Could you check a few things on this model? Use its own coordinates, in mm. A direction names the side the tool comes from. Coordinates: 2 decimals unless noted, no trailing zeros. Write each loop counter-clockwise with the first axis right and the second up, starting at its lowest first coordinate (ties: lowest second). Pieces come first, ordered by that corner, then holes.
```python
from build123d import *

# Parameters (mm, degrees)
ESQUISSE1_R          = 1
BASE_EXTRUSION_DEPTH = 1.2


with BuildPart() as part:
    # Esquisse1 → Base-Extrusion (new body)
    with BuildSketch(Plane.XY):
        with BuildLine():
            Line((-1, -11.406248288), (-1, -15.467708298))
            ThreePointArc((-1, -15.467708298), (-2.37520157, -15.316932379), (-3.731481481, -15.044136597))
            ThreePointArc((-3.731481481, -15.044136597), (-4.825271875, -14.335239515), (-5.25, -13.102957681))
            Line((-5.25, -13.102957681), (-5.25, -12.716407865))
            ThreePointArc((-5.25, -12.716407865), (-5.532204997, -11.692112826), (-6.299180328, -10.956878965))
            ThreePointArc((-6.299180328, -10.956878965), (0, 13.95), (6.299180328, -10.956878965))
            ThreePointArc((6.299180328, -10.956878965), (5.532204997, -11.692112826), (5.25, -12.716407865))
            Line((5.25, -12.716407865), (5.25, -13.102957681))
            ThreePointArc((5.25, -13.102957681), (4.825271875, -14.335239515), (3.731481481, -15.044136597))
            ThreePointArc((3.731481481, -15.044136597), (2.37520157, -15.316932379), (1, -15.467708298))
            Line((1, -15.467708298), (1, -11.406248288))
            ThreePointArc((1, -11.406248288), (0, 11.45), (-1, -11.406248288))
        make_face()
        with Locations((3.25, -13.102957681)):
            Circle(ESQUISSE1_R, mode=Mode.SUBTRACT)
        with Locations((-3.25, -13.102957681)):
            Circle(ESQUISSE1_R, mode=Mode.SUBTRACT)
    extrude(amount=BASE_EXTRUSION_DEPTH)


solid = part.part
```
1. I want a section at A-A on z = 0.4. Please give me the cut outline in (x, y), plus the area to 3 significant figures.
Verdict:
outline: (-6.3, -10.96) arc R2 cw to (-5.25, -12.72) - (-5.25, -13.1) arc R2 ccw to (-3.73, -15.04) arc R15.5 ccw to (-1, -15.47) - (-1, -11.41) arc R11.45 cw (long way) to (1, -11.41) - (1, -15.47) arc R15.5 ccw to (3.73, -15.04) arc R2 ccw to (5.25, -13.1) - (5.25, -12.72) arc R2 cw to (6.3, -10.96) arc R13.25 ccw (long way) to start; hole circle Ø2 at (-3.25, -13.1); hole circle Ø2 at (3.25, -13.1)
area: 156 mm2
2. If we mould it in two halves opening along X, with no side actions, what happens to faces 1 (the face through (1, -13, 1)), 2 (the face through (-3.38, -12.11, 0.59)), 3 (the face through (-2.36, -15.32, 0.59)), 4 (the face through (2.394, -15.314, 0.592))? For each: pulls with the +X half, pulls with the -X half, needs draft (parallel to the pull), parting line crosses it, or undercut.
Verdict:
face 1: undercut
face 2: undercut
face 3: pulls with the -X half
face 4: pulls with the +X half
3. I want a section at D-D on x = -3.25. Please give me the cut outline in (y, z).
Verdict:
outline: (-15.16, 0) - (-14.1, 0) - (-14.1, 1.2) - (-15.16, 1.2) - close; (-12.1, 0) - (-10.98, 0) - (-10.98, 1.2) - (-12.1, 1.2) - close; (10.98, 0) - (13.55, 0) - (13.55, 1.2) - (10.98, 1.2) - close
4. I want a section at C-C on x = 8.75. Please give me the cut outline in (y, z).
Verdict:
outline: (-9.25, 0) - (-7.39, 0) - (-7.39, 1.2) - (-9.25, 1.2) - close; (7.39, 0) - (10.65, 0) - (10.65, 1.2) - (7.39, 1.2) - close
5. For pin 1 (10 mm diameter, centred on x = 3.5, y = -4.5, fed in from -Z); pin 2 (2.5 mm diameter, centred on x = 3.25, y = -13.1, fed in from -Z); pin 3 (0.6 mm diameter, centred on y = -13, z = 0.5, fed in from -X), each with a flat end and sliding along its axis, tell me the tip position at first contact or that it passes through.
Verdict:
pin 1: passes through
pin 2: stops at z = 0
pin 3: stops at x = -5.25
6. I want a section at B-B on y = 4.75. Please give me the cut outline in (x, z), plus the area to 3 significant figures.
Verdict:
outline: (-12.62, 0) - (-10.42, 0) - (-10.42, 1.2) - (-12.62, 1.2) - close; (10.42, 0) - (12.62, 0) - (12.62, 1.2) - (10.42, 1.2) - close
area: 5.27 mm2
7. On a 3-axis mill with a long thin cutter (end or side, diameter ignored), from which of +Z, -Z, +X, -X, +Y, -Y can I reach the whole of each face in a straight line? I mean faces 5 (the face through (-2.9, 11.3, 1.2)), 6 (the face through (-1, -13, 1)). Say none if no direction works.
Verdict:
face 5: +Z, +X, -X, +Y, -Y
face 6: +Z, -Z, -Y
8. Please list where these lines run through material, in increasing order: line 1 along Y through (x, z) = (-2.5, 0.75); line 2 along Y through (x, z) = (-3.25, 0.6); line 3 along Y through (x, z) = (7.75, 0.75).
Verdict:
line 1: y = -15.3 to -13.76, -12.44 to -11.17, 11.17 to 13.71
line 2: y = -15.16 to -14.1, -12.1 to -10.98, 10.98 to 13.55
line 3: y = -10.05 to -8.43, 8.43 to 11.45
